Verification items for this drawing (mm, ordinates from the low corner). Round coordinates to 2 decimals unless told otherwise and drop trailing zeros. Write each loop counter-clockwise with the first axis right and the second up, starting at its lowest first coordinate (ties: lowest second). Pieces come first, ordered by that corner, then holes.
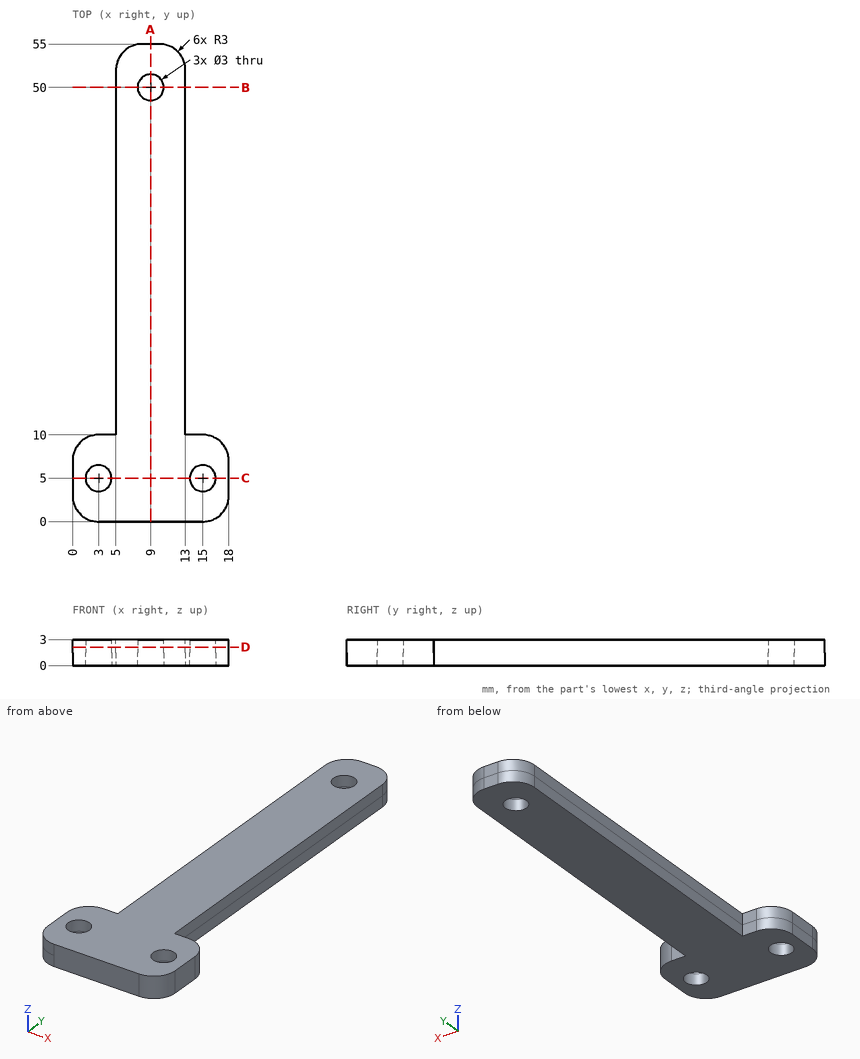
1. Depth check by flat-ended pin: pin 1 Ø1.6 at (x, z) = (14, 1.5) entering from +Y; pin 2 Ø4 at (x, y) = (15, 5) entering from +Z; pin 3 Ø0.8 at (y, z) = (35.5, 2.5) entering from +X; pin 4 Ø1.6 at (y, z) = (35, 0.5) entering from -X. Enter the tip coordinate at first touch or a pass-through.
2. Scan lines: line 1 along X through (y, z) = (44.5, 0.15); line 2 along X through (y, z) = (49, 2.45); line 3 along Y through (x, z) = (14, 1.5). Record each from-to range of solid material in increasing order.
3. Section check B-B (y = 50). Record the cut outline in (x, z).
4. Section check A-A (x = 9). Record the cut outline in (y, z), plus the area to 3 significant figures.
5. Section check C-C (y = 5). Record the cut outline in (x, z), plus the area to 3 significant figures.
6. Section check D-D (z = 2.15). Record the cut outline in (x, y).
Results below:
1. pin 1: stops at y = 10
1. pin 2: stops at z = 3
1. pin 3: stops at x = 13
1. pin 4: stops at x = 5
2. line 1: x = 5 to 13
2. line 2: x = 5 to 7.88, 10.12 to 13
2. line 3: y = 0 to 3.88, 6.12 to 10
3. outline: (5, 0) - (7.5, 0) - (7.5, 3) - (5, 3) - close; (10.5, 0) - (13, 0) - (13, 3) - (10.5, 3) - close
4. outline: (0, 0) - (48.5, 0) - (48.5, 3) - (0, 3) - close; (51.5, 0) - (55, 0) - (55, 3) - (51.5, 3) - close
4. area: 156 mm2
5. outline: (0, 0) - (1.5, 0) - (1.5, 3) - (0, 3) - close; (4.5, 0) - (13.5, 0) - (13.5, 3) - (4.5, 3) - close; (16.5, 0) - (18, 0) - (18, 3) - (16.5, 3) - close
5. area: 36.0 mm2
6. outline: (0, 3) arc R3 ccw to (3, 0) - (15, 0) arc R3 ccw to (18, 3) - (18, 7) arc R3 ccw to (15, 10) - (13, 10) - (13, 52) arc R3 ccw to (10, 55) - (8, 55) arc R3 ccw to (5, 52) - (5, 10) - (3, 10) arc R3 ccw to (0, 7) - close; hole circle Ø3 at (3, 5); hole circle Ø3 at (9, 50); hole circle Ø3 at (15, 5)
